from build123d import *

# Parameters (mm, degrees)
SKETCH1_R           = 27.5
SKETCH1_R_2         = 16
BOSS_EXTRUDE1_DEPTH = 12
SKETCH1_2_R         = 16
BOSS_EXTRUDE2_DEPTH = 44.2
SKETCH3_R           = 8.3
SKETCH3_R_2         = 3.9
CUT_EXTRUDE1_DEPTH  = 45.2


with BuildPart() as part:
    # Sketch1 → Boss-Extrude1 (new body)
    with BuildSketch(Plane(origin=(0, 0, 0), x_dir=(1, 0, 0), z_dir=(0, 1, 0))):
        Circle(SKETCH1_R)
        Circle(SKETCH1_R_2, mode=Mode.SUBTRACT)
    extrude(amount=BOSS_EXTRUDE1_DEPTH)

    # Sketch1<2> → Boss-Extrude2 (add)
    with BuildSketch(Plane(origin=(0, 0, 0), x_dir=(1, 0, 0), z_dir=(0, 1, 0))):
        Circle(SKETCH1_2_R)
    extrude(amount=BOSS_EXTRUDE2_DEPTH)

    # Sketch3 → Cut-Extrude1 (cut, through all)
    with BuildSketch(Plane(origin=(0, 0, 0), x_dir=(1, 0, 0), z_dir=(0, 1, 0))):
        Circle(SKETCH3_R)
        with Locations((0, -21.869969165)):
            Circle(SKETCH3_R_2)
        with Locations((-18.939948877, -10.934984583)):
            Circle(SKETCH3_R_2)
        with Locations((-18.939948877, 10.934984583)):
            Circle(SKETCH3_R_2)
        with Locations((0, 21.869969165)):
            Circle(SKETCH3_R_2)
        with Locations((18.939948877, 10.934984583)):
            Circle(SKETCH3_R_2)
        with Locations((18.939948877, -10.934984583)):
            Circle(SKETCH3_R_2)
    extrude(amount=CUT_EXTRUDE1_DEPTH, mode=Mode.SUBTRACT)


solid = part.part
Input: part model. Units: mm. Frame: model coordinates. Give positions to 0.01 mm unless a question says otherwise; leave off trailing zeros. Order: outer loops, then holes, each group sorted by start corner. A loop starts at its lowest first (then second) coordinate and runs counter-clockwise, first axis right, second up. Notation, with made-up numbers: (-13, 83.5) - (0, 83.5) arc R18 ccw to (0, 97.5) - close; hole circle Ø2 at (-17, 26). An arc over 180 degrees is marked (long way). Answer as a JSON object with one key per item and string values. Group by question number.
Q1. Cut plane B-B, the plane x = 0. Output: boundary loops of the cut face in (y, z).
Q2. Cut plane C-C, the plane x = 7. Output: boundary loops of the cut face in (y, z), then the cut area to 3 significant figures.
Q3. Line query: probe 1 along Z at (x, y) = (0, 3.75); probe 2 along Z at (x, y) = (0, 32.5); probe 3 along Y at (x, z) = (-20, -17). Output: solid intervals per line, ascending.
Q4. Cut plane D-D, the plane y = 4.5. Output: boundary loops of the cut face in (x, z), then the cut area to 3 significant figures.
Q5. Mould query, pull axis X, two halves, no side actions, for faces 1 (the face through (-3.47, 27.87, 15.62)), 2 (the face through (18.09, 5.92, -7.13)), 3 (the face through (12, 12, 12)). Classes: pulls with the +X half, pulls with the -X half, needs draft (parallel to the pull), parting line crosses it, or undercut.
Q6. Cut plane A-A, the plane z = 0. Output: boundary loops of the cut face in (x, y), then the cut area to 3 significant figures.
Q7. First-contact query: pin 1 Ø5 at (x, y) = (0, 35) entering from +Z; pin 2 Ø7 at (x, z) = (0, 21.87) entering from -Y; pin 3 Ø8 at (y, z) = (11, -9.5) entering from -X; pin 4 Ø10 at (x, z) = (0, -21.87) entering from +Y. Flat tips, straight axial feed; report the tip coordinate or a pass-through.
Results:
{
 "1": {"outline": "(0, -27.5) - (12, -27.5) - (12, -25.77) - (0, -25.77) - close; (0, -17.97) - (12, -17.97) - (12, -16) - (44.2, -16) - (44.2, -8.3) - (0, -8.3) - close; (0, 8.3) - (44.2, 8.3) - (44.2, 16) - (12, 16) - (12, 17.97) - (0, 17.97) - close; (0, 25.77) - (12, 25.77) - (12, 27.5) - (0, 27.5) - close"},
 "2": {"outline": "(0, -26.59) - (12, -26.59) - (12, -14.39) - (44.2, -14.39) - (44.2, -4.46) - (0, -4.46) - close; (0, 4.46) - (44.2, 4.46) - (44.2, 14.39) - (12, 14.39) - (12, 26.59) - (0, 26.59) - close", "area": "1,170 mm^2"},
 "3": {"probe 1": "-27.5 to -25.77, -17.97 to -8.3, 8.3 to 17.97, 25.77 to 27.5", "probe 2": "-16 to -8.3, 8.3 to 16", "probe 3": "0 to 12"},
 "4": {"outline": "circle Ø55 at (0, 0); hole circle Ø7.8 at (-18.94, -10.93); hole circle Ø7.8 at (-18.94, 10.93); hole circle Ø16.6 at (0, 0); hole circle Ø7.8 at (0, -21.87); hole circle Ø7.8 at (0, 21.87); hole circle Ø7.8 at (18.94, -10.93); hole circle Ø7.8 at (18.94, 10.93)", "area": "1,870 mm^2"},
 "5": {"face 1": "parting line crosses it", "face 2": "undercut", "face 3": "needs draft"},
 "6": {"outline": "(-27.5, 0) - (-8.3, 0) - (-8.3, 44.2) - (-16, 44.2) - (-16, 12) - (-27.5, 12) - close; (8.3, 0) - (27.5, 0) - (27.5, 12) - (16, 12) - (16, 44.2) - (8.3, 44.2) - close", "area": "957 mm^2"},
 "7": {"pin 1": "z = 16", "pin 2": "through", "pin 3": "x = -26.94", "pin 4": "y = 12"}
}
